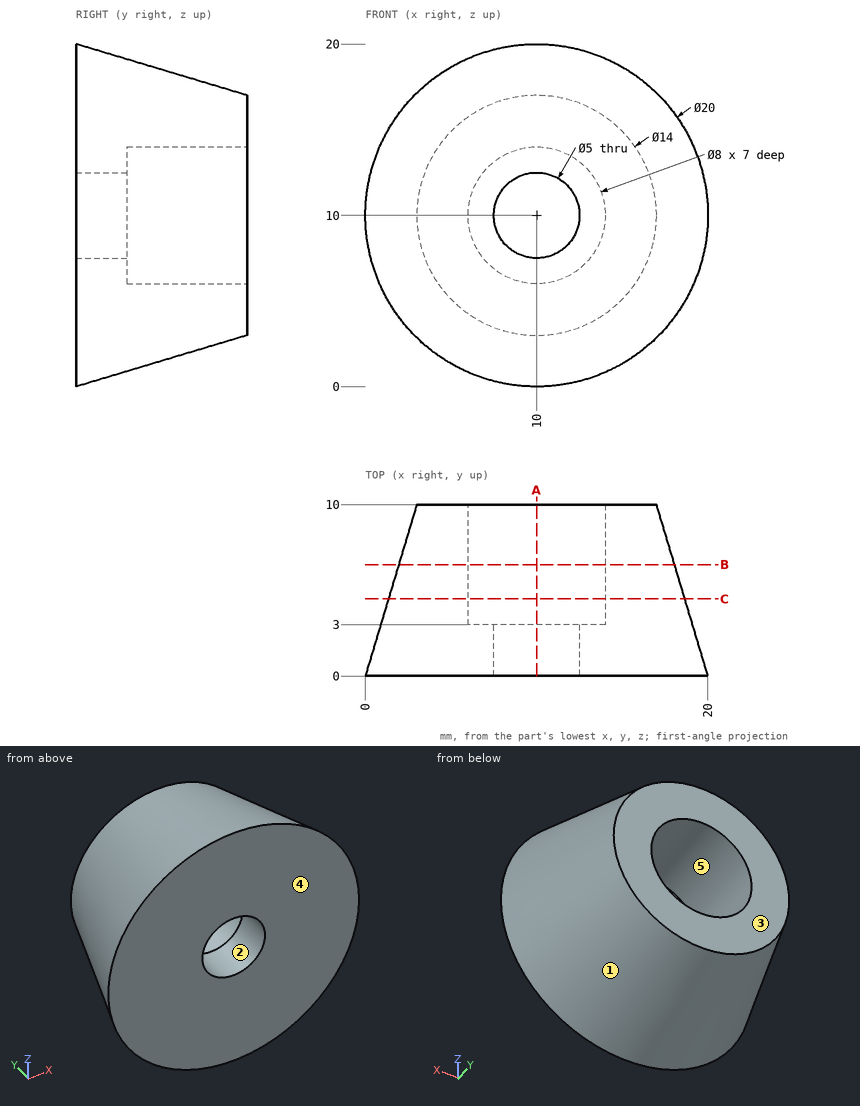
Drawing for the job (mm, zero at the part's lowest x, y, z). A direction names the side the tool comes from. Coordinates: 2 decimals unless noted, no trailing zeros. Write each loop counter-clockwise with the first axis right and the second up, starting at its lowest first coordinate (ties: lowest second). Pieces come first, ordered by that corner, then holes. Notation, with made-up numbers: (-40, -32) -> (-11, -32) arc R19 ccw to (-11, -6) -> close; hole circle Ø5 at (-3, 40.25). An arc over 180 degrees is marked (long way). One line per item, written item: value. Start each with the question number.
1) Slice it at A-A on x = 10. Write the cut outline in (y, z), then the cut area to 3 significant figures.
2) Slice it at C-C on y = 4.5. Write the cut outline in (x, z), then the cut area to 3 significant figures.
3) Which spindle directions (+Z, -Z, +X, -X, +Y, -Y) get a long thin tool onto all of the face, cutting with end or side? Do the marked faces 4 and 5. Say none if no direction does.
4) Probe probe 1 along Z at (x, y) = (10, 1.9); probe 2 along X at (y, z) = (4, 7.5); probe 3 along Z at (x, y) = (10, 1.75) (3 decimals). List the from-to ranges inside material, lowest first.
5) Pull direction X, two halves, no side cores. Call the marked faces 1, 2 and 3: +X half, -X half, draft (parallel to the pull), parting line (faces both ways), or undercut.
6) Slice it at B-B on y = 6.5. Write the cut outline in (x, z), then the cut area to 3 significant figures.
7) Flat gauge pins, fed straight in: pin 1 Ø3 at (y, z) = (7, 6) entering from +X; pin 2 Ø2 at (y, z) = (2, 5.5) entering from -X; pin 3 Ø7 at (x, z) = (10, 10) entering from +Y. Where does each tip first touch, or does it go through?
Answers follow:
1. outline: (0, 0) -> (10, 3) -> (10, 6) -> (3, 6) -> (3, 7.5) -> (0, 7.5) -> close; (0, 12.5) -> (3, 12.5) -> (3, 14) -> (10, 14) -> (10, 17) -> (0, 20) -> close
1. area: 99.0 mm2
2. outline: circle Ø17.3 at (10, 10); hole circle Ø8 at (10, 10)
2. area: 185 mm2
3. face 4: +Z, -Z, +X, -X, -Y
3. face 5: +Y
4. probe 1: 0.57 to 7.5, 12.5 to 19.43
4. probe 2: 1.56 to 6.88, 13.12 to 18.44
4. probe 3: 0.525 to 7.5, 12.5 to 19.475
5. face 1: parting line
5. face 2: undercut
5. face 3: draft
6. outline: circle Ø16.1 at (10, 10); hole circle Ø8 at (10, 10)
6. area: 153 mm2
7. pin 1: x = 17.68
7. pin 2: x = 1.16
7. pin 3: y = 3
